from build123d import *

# Parameters (mm, degrees)
SKETCH1_W           = 200
SKETCH1_H           = 1200
BOSS_EXTRUDE1_DEPTH = 5
CUT_EXTRUDE1_DEPTH  = 609.296802556
SKETCH5_W           = 60
SKETCH5_H           = 1000
CUT_EXTRUDE3_DEPTH  = 609.296802556
FILLET2_R           = 5
SKETCH6_R           = 3
CUT_EXTRUDE4_DEPTH  = 609.296802556
FILLET3_R           = 2
SKETCH9_R           = 2.1
CUT_EXTRUDE5_DEPTH  = 609.296802556


with BuildPart() as part:
    # Sketch1 → Boss-Extrude1 (new body)
    with BuildSketch(Plane.XY):
        Rectangle(SKETCH1_W, SKETCH1_H)
    extrude(amount=BOSS_EXTRUDE1_DEPTH)

    # Sketch3 → Cut-Extrude1 (cut, through all)
    with BuildSketch(Plane.XY.offset(5)):
        with BuildLine():
            Line((-100, -600), (-100, -564.197190267))
            ThreePointArc((-100, -564.197190267), (-74.683590452, -574.683590452), (-64.197190267, -600))
            Line((-64.197190267, -600), (-100, -600))
        make_face()
        with BuildLine():
            Line((64.197190267, -600), (100, -600))
            Line((100, -600), (100, -564.197190267))
            ThreePointArc((100, -564.197190267), (74.683590452, -574.683590452), (64.197190267, -600))
        make_face()
    extrude(amount=-CUT_EXTRUDE1_DEPTH, mode=Mode.SUBTRACT)

    # Sketch5 → Cut-Extrude3 (cut, through all)
    with BuildSketch(Plane.XY.offset(5)):
        Rectangle(SKETCH5_W, SKETCH5_H)
    extrude(amount=-CUT_EXTRUDE3_DEPTH, mode=Mode.SUBTRACT)

    # Fillet2
    fillet2_edges = [part.edges().sort_by_distance(p)[0] for p in [
        (30, 500, 2.5),
        (30, -500, 2.5),
        (-30, -500, 2.5),
        (-30, 500, 2.5),
    ]]
    fillet(fillet2_edges, radius=FILLET2_R)

    # Sketch6 → Cut-Extrude4 (cut, through all)
    with BuildSketch(Plane.XY.offset(5)):
        with Locations((83.193225438, -34)):
            Circle(SKETCH6_R)
        with Locations((83.193225438, 34)):
            Circle(SKETCH6_R)
        with Locations(Location((-83.193225438, 34, 0), (0, 0, 180))):
            Circle(SKETCH6_R)
        with Locations(Location((-83.193225438, -34, 0), (0, 0, 180))):
            Circle(SKETCH6_R)
    extrude(amount=-CUT_EXTRUDE4_DEPTH, mode=Mode.SUBTRACT)

    # Fillet3
    fillet3_edges = [part.edges().sort_by_distance(p)[0] for p in [
        (64.197190267, -600, 2.5),
        (100, -564.197190267, 2.5),
        (-64.197190267, -600, 2.5),
        (-100, -564.197190267, 2.5),
        (-100, 600, 2.5),
        (100, 600, 2.5),
    ]]
    fillet(fillet3_edges, radius=FILLET3_R)

    # Sketch9 → Cut-Extrude5 (cut, through all)
    with BuildSketch(Plane.XY.offset(5)):
        with Locations((-40, 550)):
            Circle(SKETCH9_R)
        with Locations((-40, 500)):
            Circle(SKETCH9_R)
        with Locations((-40, 450)):
            Circle(SKETCH9_R)
        with Locations((-40, 400)):
            Circle(SKETCH9_R)
        with Locations((-40, 350)):
            Circle(SKETCH9_R)
        with Locations((-40, 300)):
            Circle(SKETCH9_R)
        with Locations((-40, 250)):
            Circle(SKETCH9_R)
        with Locations((-40, 200)):
            Circle(SKETCH9_R)
        with Locations((-40, 150)):
            Circle(SKETCH9_R)
        with Locations((-40, 100)):
            Circle(SKETCH9_R)
        with Locations((-40, 50)):
            Circle(SKETCH9_R)
        with Locations((-40, 0)):
            Circle(SKETCH9_R)
        with Locations((-40, -50)):
            Circle(SKETCH9_R)
        with Locations((-40, -100)):
            Circle(SKETCH9_R)
        with Locations((-40, -150)):
            Circle(SKETCH9_R)
        with Locations((-40, -200)):
            Circle(SKETCH9_R)
        with Locations((-40, -250)):
            Circle(SKETCH9_R)
        with Locations((-40, -300)):
            Circle(SKETCH9_R)
        with Locations((-40, -350)):
            Circle(SKETCH9_R)
        with Locations((-40, -400)):
            Circle(SKETCH9_R)
        with Locations((-40, -450)):
            Circle(SKETCH9_R)
        with Locations((-40, -500)):
            Circle(SKETCH9_R)
        with Locations((-40, -550)):
            Circle(SKETCH9_R)
    cut_extrude5 = extrude(amount=-CUT_EXTRUDE5_DEPTH, mode=Mode.SUBTRACT)

    # Mirror1: Cut-Extrude5 across plane
    add(cut_extrude5.mirror(Plane(origin=(0, 0, 0), x_dir=(0, 0, 1), z_dir=(1, 0, 0))), mode=Mode.SUBTRACT)


solid = part.part
Here's how the part is built. I have some questions about the finished solid (model axes, mm). Round coordinates to 2 decimals unless told otherwise and drop trailing zeros. Order: outer loops, then holes, each group sorted by start corner. A loop starts at its lowest first (then second) coordinate and runs counter-clockwise, first axis right, second up. Notation, with made-up numbers: M 84.25,-27.5 L 142.25,-27.5 A28 cw 142.25,0.5 Z; hole C -29,56.5 d9. An arc over 180 degrees is marked long. Return JSON: item names as keys, results as strings. Group by question number.
1. If we section it at B-B on z = 2.5: State how many separate pieces and enclosed holes the cut face has, then the cut area to 3 significant figures.
2. If we section it at A-A on y = 81.5: List the corners of the cut face in (x, z) for me, then the cut area to 3 significant figures.
3. Please list where these lines run through material, in increasing order: probe 1 along X at (y, z) = (150, 1.2); probe 2 along X at (y, z) = (-228, 0.65); probe 3 along Y at (x, z) = (-21.5, 2.3).
Reply:
{
 "1": {"separate pieces": "1", "enclosed holes": "51", "area": "177,000 mm^2"},
 "2": {"outline": "M -100,0 L -30,0 L -30,5 L -100,5 Z; M 30,0 L 100,0 L 100,5 L 30,5 Z", "area": "700 mm^2"},
 "3": {"probe 1": "-100 to -42.1, -37.9 to -30, 30 to 37.9, 42.1 to 100", "probe 2": "-100 to -30, 30 to 100", "probe 3": "-600 to -500, 500 to 600"}
}
